The model under review builds one solid part; all positions refer to its coordinate system, in mm. A direction names the side the tool comes from. Coordinates: 2 decimals unless noted, no trailing zeros. Loops run counter-clockwise (first coordinate to the right, second up) from the corner with the lowest first, then second, coordinate; pieces in that order, holes last. Notation, with made-up numbers: M 56,34.5 L 84,34.5 A17 ccw 84,46.5 Z; hole C 21,-5.5 d7. An arc over 180 degrees is marked long. One line per item, written item: value.
```python
from build123d import *

# Parameters (mm, degrees)
SKETCH1_W           = 6
SKETCH1_H           = 10.023203152
BOSS_EXTRUDE1_DEPTH = 3
SKETCH1_3_W         = 4
SKETCH1_3_H         = 10.023203152
BOSS_EXTRUDE2_DEPTH = 19.05
SKETCH2_R           = 1.5875
CUT_EXTRUDE1_DEPTH  = 19.05
SKETCH3_W           = 80.796379589
SKETCH3_H           = 10
BOSS_EXTRUDE3_DEPTH = 3


with BuildPart() as part:
    # Sketch1 → Boss-Extrude1 (new body)
    with BuildSketch(Plane(origin=(0, 0, 0), x_dir=(1, 0, 0), z_dir=(0, 1, 0))):
        Polygon((0, 50.8), (0, 0), (50.8, 0), (50.8, 50.8), (32.4, 50.8), (28.4, 50.8), (22.4, 50.8), (18.4, 50.8), align=None)
        with Locations((25.4, 55.811601576)):
            Rectangle(SKETCH1_W, SKETCH1_H)
    extrude(amount=BOSS_EXTRUDE1_DEPTH)

    # Sketch1_3 → Boss-Extrude2 (add)
    with BuildSketch(Plane(origin=(0, 0, 0), x_dir=(1, 0, 0), z_dir=(0, 1, 0))):
        with Locations((30.4, 55.811601576)):
            Rectangle(SKETCH1_3_W, SKETCH1_3_H)
        with Locations((20.4, 55.811601576)):
            Rectangle(SKETCH1_3_W, SKETCH1_3_H)
    extrude(amount=BOSS_EXTRUDE2_DEPTH)

    # Sketch2 → Cut-Extrude1 (cut)
    with BuildSketch(Plane(origin=(32.4, 0, 0), x_dir=(0, 0, -1), z_dir=(1, 0, 0))):
        with Locations((55.811601576, 14.038398424)):
            Circle(SKETCH2_R)
        with BuildLine():
            Line((50.8, 14.038398424), (49.911458456, 20.395059664))
            Line((49.911458456, 20.395059664), (64.501767063, 21.247740037))
            Line((64.501767063, 21.247740037), (60.823203152, 14.038398424))
            ThreePointArc((60.823203152, 14.038398424), (55.811601576, 19.05), (50.8, 14.038398424))
        make_face()
    extrude(amount=-CUT_EXTRUDE1_DEPTH, mode=Mode.SUBTRACT)

    # Sketch3 → Boss-Extrude3 (add)
    with BuildSketch(Plane.XZ):
        Polygon((0, 0), (-30, 0), (-30, -10), (50.8, -10), (50.8, 0), align=None)
        with Locations((10.398189795, -29.723216131)):
            Rectangle(SKETCH3_W, SKETCH3_H)
    extrude(amount=BOSS_EXTRUDE3_DEPTH)


solid = part.part
```
(1) Tool access review of faces 4 (the face through (25, 0, -36)), 5 (the face through (10, -1, -34.723)), 6 (the face through (9, 1, -50.8)), 7 (the face through (22.4, 11, -56)): name each direction out of +Z, -Z, +X, -X, +Y, -Y from which nothing blocks a thin tool from reaching the whole face with its end or side.
Checks:
face 4: +X, -X, -Y
face 5: -Z, +X, -X, -Y
face 6: -Z, -X, +Y, -Y
face 7: +Z, -Z, +Y
(2) Draft analysis for pull direction Z (two halves, no side actions). For faces 1 (the face through (42, 1, -50.8)), 2 (the face through (10, -1, -24.723)), 3 (the face through (-15, 0, -30)), state which applies: pulls with the +Z half, pulls with the -Z half, needs draft (parallel to the pull), parting line crosses it, or undercut.
Checks:
face 1: pulls with the -Z half
face 2: undercut
face 3: needs draft
(3) Add section B-B on x = 40.5. State the section outline as (y, z) points, then the cut area to 3 significant figures.
Checks:
outline: M -3,-34.72 L 0,-34.72 L 0,-50.8 L 3,-50.8 L 3,0 L -3,0 L -3,-10 L 0,-10 L 0,-24.72 L -3,-24.72 Z
area: 212 mm^2
(4) Insertion check: pin 1 Ø8 at (x, z) = (-14.5, -29.5) entering from +Y; pin 2 Ø0.9 at (y, z) = (2, -15) entering from -X; pin 3 Ø4 at (x, z) = (0.5, -22.5) entering from -Y; pin 4 Ø3.5 at (x, y) = (5, -2) entering from +Z. Each pin has a flat end and moves straight along its axis. Give the tip position at first contact, or say it passes through.
Checks:
pin 1: y = 0
pin 2: x = 0
pin 3: y = 0
pin 4: z = 0
(5) Add section A-A on y = 9.5. State the section outline as (x, z) points.
Checks:
outline: M 18.4,-60.82 L 22.4,-60.82 L 22.4,-50.8 L 18.4,-50.8 Z; M 28.4,-60.82 L 32.4,-60.82 L 32.4,-50.8 L 28.4,-50.8 Z
(6) Add section D-D on y = 1.5. State the section outline as (x, z) points.
Checks:
outline: M 0,-50.8 L 18.4,-50.8 L 18.4,-60.82 L 32.4,-60.82 L 32.4,-50.8 L 50.8,-50.8 L 50.8,0 L 0,0 Z
(7) To check wall thickness, follow L1, parallel to Z at x = 12.5, y = -0.5; L2, parallel to Y at x = 44.5, z = -18; L3, parallel to Y at x = 24, z = -5.5. State the ranges of each line that lie inside material, in increasing order. Write a range as [from, to].
Checks:
L1: [-34.72, -24.72], [-10, 0]
L2: [0, 3]
L3: [-3, 3]
